Check sheet for the drawn part. Datum: minimum x, y, z corner. Units: mm. A direction names the side the tool comes from. Give positions to 0.01 mm unless a question says otherwise; leave off trailing zeros. Loops run counter-clockwise (first coordinate to the right, second up) from the corner with the lowest first, then second, coordinate; pieces in that order, holes last. Notation, with made-up numbers: (30, -12) - (84, -12) arc R25 cw to (84, 26) - close; hole circle Ø10 at (5, 9.5). An arc over 180 degrees is marked (long way). Use one line per item in the form item = value.
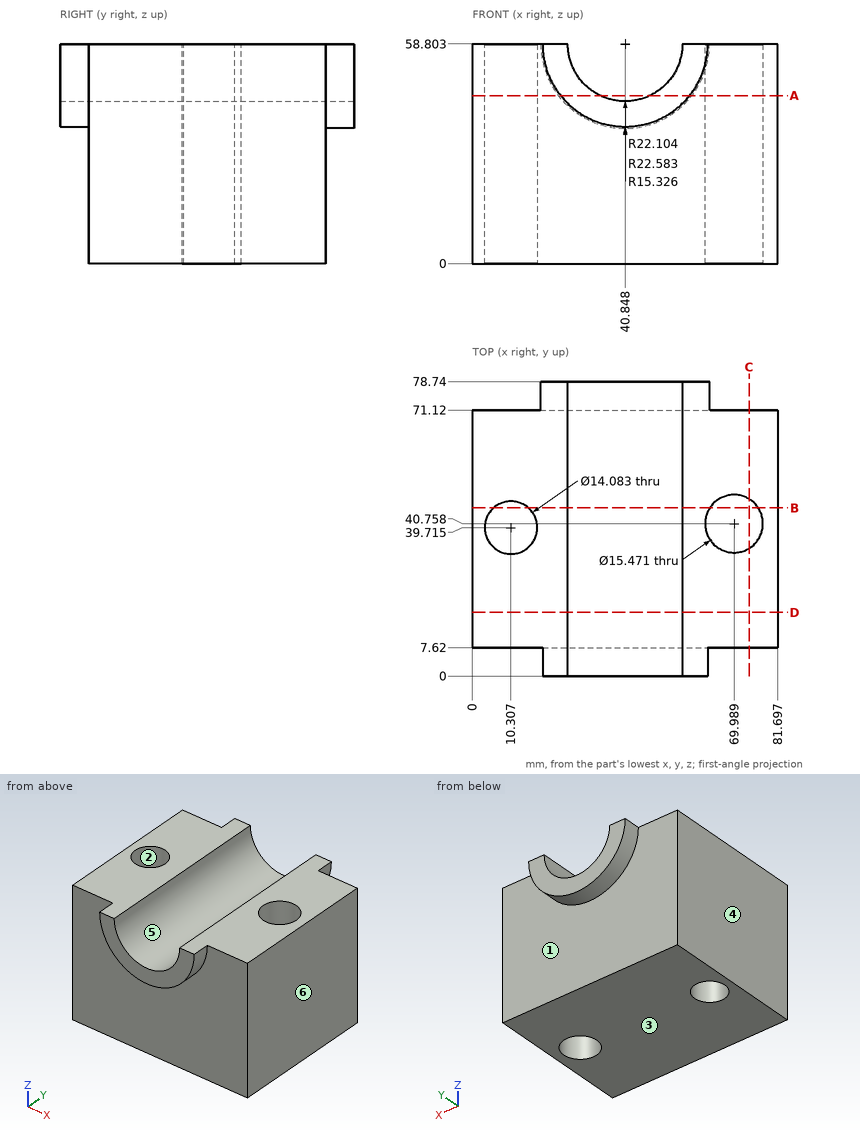
1. Scan lines: probe 1 along X at (y, z) = (40, 13); probe 2 along X at (y, z) = (39, 2.5) (1 decimal); probe 3 along Y at (x, z) = (37, 23). Record each from-to range of solid material in increasing order.
Result set:
probe_1 = 0 to 3.27, 17.34 to 62.29, 77.69 to 81.7
probe_2 = 0 to 3.3, 17.3 to 62.5, 77.5 to 81.7
probe_3 = 7.62 to 71.12
2. Depth check by flat-ended pin: pin 1 Ø12.5 at (x, y) = (69.99, 40.76) entering from +Z; pin 2 Ø17.5 at (x, z) = (55, 29) entering from -Y; pin 3 Ø1 at (x, y) = (33.5, 52.5) entering from +Z; pin 4 Ø3 at (x, z) = (33, 14) entering from +Y. Enter the tip coordinate at first touch or a pass-through.
Result set:
pin_1 = through
pin_2 = 7.62
pin_3 = 45.64
pin_4 = 71.12
3. Tool access check on the marked faces 1 and 2. Record the directions out of +Z, -Z, +X, -X, +Y, -Y that give a thin tool (end or side, any length) a straight path to the whole face; none if there is none.
Result set:
face_1 = -Z, +Y
face_2 = +Z, -Z
4. Section check C-C, the plane x = 74. Record the cut outline in (y, z), then the cut area to 3 significant figures.
Result set:
outline = (7.62, 0) - (34.14, 0) - (34.14, 58.8) - (7.62, 58.8) - close; (47.37, 0) - (71.12, 0) - (71.12, 58.8) - (47.37, 58.8) - close
area = 2,960 mm²
5. Section check D-D, the plane y = 17. Record the cut outline in (x, z) (1 decimal), then the cut area to 4 significant figures.
Result set:
outline = (0, 0) - (81.7, 0) - (81.7, 58.8) - (56.2, 58.8) arc R15.3 cw to (25.5, 58.8) - (0, 58.8) - close
area = 4,435 mm²
6. Section check B-B, the plane y = 45. Record the cut outline in (x, z) (1 decimal), then the cut area to 3 significant figures.
Result set:
outline = (0, 0) - (5.7, 0) - (5.7, 58.8) - (0, 58.8) - close; (15, 0) - (63.5, 0) - (63.5, 58.8) - (56.2, 58.8) arc R15.3 cw to (25.5, 58.8) - (15, 58.8) - close; (76.5, 0) - (81.7, 0) - (81.7, 58.8) - (76.5, 58.8) - close
area = 3,130 mm²
7. Section check A-A, the plane z = 45. Record the cut outline in (x, y) (1 decimal), then the cut area to 3 significant figures.
Result set:
outline = (0, 7.6) - (23.6, 7.6) - (23.6, 0) - (34.2, 0) - (34.2, 78.7) - (23, 78.7) - (23, 71.1) - (0, 71.1) - close; (47.5, 0) - (58.1, 0) - (58.1, 7.6) - (81.7, 7.6) - (81.7, 71.1) - (58.7, 71.1) - (58.7, 78.7) - (47.5, 78.7) - close; hole circle Ø14.1 at (10.3, 39.7); hole circle Ø15.5 at (70, 40.8)
area = 4,330 mm²
8. Draft check along X on the marked faces 3, 4, 5 and 6. Enter one of: released by +X, released by -X, zero draft, split by the parting line, or undercut.
Result set:
face_3 = zero draft
face_4 = released by -X
face_5 = undercut
face_6 = released by +X
